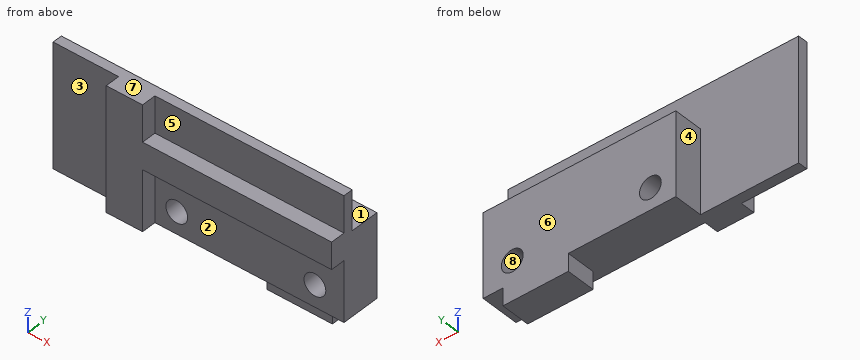
from build123d import *

# Parameters (mm, degrees)
SKETCH_1_W          = 40
SKETCH_1_H          = 17
EXTRUDE_1_DEPTH     = 1.33
SKETCH_2_W          = 9
SKETCH_2_H          = 2.4
EXTRUDE_2_DEPTH     = 4
SKETCH_3_W          = 26
SKETCH_3_H          = 3.69
EXTRUDE_3_DEPTH     = 2
SKETCH_4_R          = 1.5
CUT_EXTRUDE_1_DEPTH = 24.392710403


with BuildPart() as part:
    # Эскиз1 → Бобышка-Вытянуть1 (new body)
    with BuildSketch(Plane(origin=(0, 0, 0), x_dir=(1, 0, 0), z_dir=(0, 1, 0))):
        Rectangle(SKETCH_1_W, SKETCH_1_H)
    extrude(amount=EXTRUDE_1_DEPTH)

    # Эскиз2 → Бобышка-Вытянуть2 (add)
    with BuildSketch(Plane(origin=(0, 1.33, 0), x_dir=(1, 0, 0), z_dir=(0, 1, 0))):
        Polygon((20, -3), (20, 8.5), (17.28, 8.5), (8.28, 8.5), (-6.5, 8.5), (-6.5, -3), align=None)
        with Locations((12.78, 9.7)):
            Rectangle(SKETCH_2_W, SKETCH_2_H)
    extrude(amount=EXTRUDE_2_DEPTH)

    # Эскиз3 → Бобышка-Вытянуть3 (add)
    with BuildSketch(Plane.XZ):
        Polygon((-11, -8.5), (-6, -8.5), (-6, -0.19), (-6, 3.5), (-6, 8.5), (-11, 8.5), align=None)
        with Locations((7, 1.655)):
            Rectangle(SKETCH_3_W, SKETCH_3_H)
    extrude(amount=EXTRUDE_3_DEPTH)

    # Эскиз4 → Вырез-Вытянуть1 (cut, through all)
    with BuildSketch(Plane.XZ):
        with Locations(Location((16, -5.5, 0), (0, 0, 270))):
            Circle(SKETCH_4_R)
        with Locations(Location((-3, -5.5, 0), (0, 0, 270))):
            Circle(SKETCH_4_R)
    extrude(amount=-CUT_EXTRUDE_1_DEPTH, mode=Mode.SUBTRACT)


solid = part.part
Model file for the job. Use its own axes, mm. Face numbers are marked on the shaded views. A direction names the side the tool comes from. Give positions to 0.01 mm unless a question says otherwise; leave off trailing zeros. Order: outer loops, then holes, each group sorted by start corner. A loop starts at its lowest first (then second) coordinate and runs counter-clockwise, first axis right, second up. Notation, with made-up numbers: (-35.75, 22) -> (13.25, 22) arc R18 ccw to (13.25, 40) -> close; hole circle Ø2 at (51.5, 47). An arc over 180 degrees is marked (long way). Use CSV: the item, a comma, the result in double quotes.
1. Band-saw the part on A-A, the plane x = 16. Give the cut face in (y, z), then the cut area to 3 significant figures.
Outcome:
outline,"(-2, -0.19) -> (0, -0.19) -> (0, -4) -> (5.33, -4) -> (5.33, 3) -> (1.33, 3) -> (1.33, 8.5) -> (0, 8.5) -> (0, 3.5) -> (-2, 3.5) -> close; (0, -8.5) -> (1.33, -8.5) -> (1.33, -10.9) -> (5.33, -10.9) -> (5.33, -7) -> (0, -7) -> close"
area,"69.6 mm²"
2. Drill centre lines: line 1 along X through (y, z) = (2.9, -5.5); line 2 along X through (y, z) = (4, -4.5); line 3 along Z through (x, y) = (14, 0.5). Where is each one in solid material? Low to high. Write a range as from..to.
Outcome:
line 1,"-6.5..-4.5, -1.5..14.5, 17.5..20"
line 2,"-6.5..-4.12, -1.88..14.88, 17.12..20"
line 3,"-8.5..8.5"
3. Band-saw the part on D-D, the plane x = 11.5. Give the cut face in (y, z).
Outcome:
outline,"(-2, -0.19) -> (0, -0.19) -> (0, -8.5) -> (1.33, -8.5) -> (1.33, -10.9) -> (5.33, -10.9) -> (5.33, 3) -> (1.33, 3) -> (1.33, 8.5) -> (0, 8.5) -> (0, 3.5) -> (-2, 3.5) -> close"
4. Drop flat-ended pins along their axis: pin 1 (1.9 mm diameter, centred on y = 3, z = -10, fed in from +X); pin 2 (4 mm diameter, centred on x = -9, y = 0, fed in from -Z); pin 3 (1.2 mm diameter, centred on y = 3, z = -5, fed in from -X); pin 4 (2.5 mm diameter, centred on x = -3, z = -5.5, fed in from +Y). Give the stop position or say it passes through.
Outcome:
pin 1,"x = 17.28"
pin 2,"z = -8.5"
pin 3,"x = -6.5"
pin 4,"through"
5. Band-saw the part on C-C, the plane z = -5.5. Give the cut face in (x, y).
Outcome:
outline,"(-20, 0) -> (-11, 0) -> (-11, -2) -> (-6, -2) -> (-6, 0) -> (-4.5, 0) -> (-4.5, 5.33) -> (-6.5, 5.33) -> (-6.5, 1.33) -> (-20, 1.33) -> close; (-1.5, 0) -> (14.5, 0) -> (14.5, 5.33) -> (-1.5, 5.33) -> close; (17.5, 0) -> (20, 0) -> (20, 5.33) -> (17.5, 5.33) -> close"
6. 3-axis set-ups, long thin cutter, end or side, ignore diameter. For the marked faces 1, 2, 3, 4 and 5: which of +Z, -Z, +X, -X, +Y, -Y reach the whole face in a straight line?
Outcome:
face 1,"+Z, +X, -X, +Y"
face 2,"-Z, +X, -Y"
face 3,"+Z, -Z, -X, -Y"
face 4,"+Z, -Z, -X, +Y"
face 5,"+Z, +X, -Y"
7. Band-saw the part on B-B, the plane y = 3.75. Give the cut face in (x, z).
Outcome:
outline,"(-6.5, -8.5) -> (8.28, -8.5) -> (8.28, -10.9) -> (17.28, -10.9) -> (17.28, -8.5) -> (20, -8.5) -> (20, 3) -> (-6.5, 3) -> close; hole circle Ø3 at (-3, -5.5); hole circle Ø3 at (16, -5.5)"
8. Mould opens along Z. For the marked faces 6, 7 and 8 say: +Z half, -Z half, draft (parallel to the pull), parting line (faces both ways), or undercut.
Outcome:
face 6,"draft"
face 7,"+Z half"
face 8,"undercut"
